Source: CAD feature listing. Evaluate the final solid. Frame: model axes, mm. A direction names the side the tool comes from. Give positions to 0.01 mm unless a question says otherwise; leave off trailing zeros. Write each loop counter-clockwise with the first axis right and the second up, starting at its lowest first coordinate (ties: lowest second). Pieces come first, ordered by that corner, then holes. Notation, with made-up numbers: M 49,1.5 L 84,1.5 A28 cw 84,21.5 Z; hole C 40,41 d9. An arc over 180 degrees is marked long. Use CSV: the item, a comma, the result in double quotes. Start each with the question number.
from build123d import *

# Parameters (mm, degrees)
BOSS_EXTRUDE1_DEPTH = 6
BOSS_EXTRUDE2_START = 6
BOSS_EXTRUDE2_DEPTH = 6
BOSS_EXTRUDE3_DEPTH = 1.5
CUT_EXTRUDE3_DEPTH  = 6
CHAMFER1_SIZE       = 0.858848527
CHAMFER1_SIZE_2     = 1
CHAMFER2_SIZE       = 1


with BuildPart() as part:
    # Sketch3 → Boss-Extrude1 (new body)
    with BuildSketch(Plane.XY):
        with BuildLine():
            Line((3.263957589, 12.181255556), (-159.230871571, 55.721613803))
            ThreePointArc((-159.230871571, 55.721613803), (-167.389036276, 0), (-159.230871571, -55.721613803))
            Line((-159.230871571, -55.721613803), (-83.597968128, -35.455838404))
            Line((-83.597968128, -35.455838404), (3.263957589, -12.181255556))
            ThreePointArc((3.263957589, -12.181255556), (12.610963724, 0), (3.263957589, 12.181255556))
        make_face()
    extrude(amount=BOSS_EXTRUDE1_DEPTH)

    # Sketch3<3> → Boss-Extrude2 (add)
    with BuildSketch(Plane.XY.offset(BOSS_EXTRUDE2_START)):
        with BuildLine():
            ThreePointArc((3.263957589, -12.181255556), (12.610963724, 0), (3.263957589, 12.181255556))
            Line((3.263957589, 12.181255556), (-159.230871571, 55.721613803))
            ThreePointArc((-159.230871571, 55.721613803), (-167.389036276, 0), (-159.230871571, -55.721613803))
            Line((-159.230871571, -55.721613803), (-83.597968128, -35.455838404))
            Line((-83.597968128, -35.455838404), (3.263957589, -12.181255556))
        make_face()
        with BuildLine():
            Line((-85.282065581, -29.695433875), (-155.066564747, -48.39413407))
            ThreePointArc((-155.066564747, -48.39413407), (-161.389036276, 0), (-155.066564747, 48.39413407))
            Line((-155.066564747, 48.39413407), (-85.282065581, 29.695433875))
            ThreePointArc((-85.282065581, 29.695433875), (-89.143036276, 0), (-85.282065581, -29.695433875))
        make_face(mode=Mode.SUBTRACT)
        with BuildLine():
            Line((1.711043318, -6.385700598), (-79.486479098, -28.142511157))
            ThreePointArc((-79.486479098, -28.142511157), (-83.143036276, 0), (-79.486479098, 28.142511157))
            Line((-79.486479098, 28.142511157), (1.711043318, 6.385700598))
            ThreePointArc((1.711043318, 6.385700598), (6.610963724, 0), (1.711043318, -6.385700598))
        make_face(mode=Mode.SUBTRACT)
    extrude(amount=BOSS_EXTRUDE2_DEPTH)

    # Sketch4 → Boss-Extrude3 (add)
    with BuildSketch(Plane.XY.offset(6)):
        with BuildLine():
            ThreePointArc((-79.486479098, 28.142511157), (-80.363791639, 24.584864194), (-81.12226241, 21))
            Line((-81.12226241, 21), (-52.830264568, 21))
            Line((-52.830264568, 21), (-79.486479098, 28.142511157))
        make_face()
        with BuildLine():
            Line((-79.486479098, -28.142511157), (-52.830264568, -21))
            Line((-52.830264568, -21), (-81.12226241, -21))
            ThreePointArc((-81.12226241, -21), (-80.363791639, -24.584864194), (-79.486479098, -28.142511157))
        make_face()
        with BuildLine():
            Line((-48.09821376, 19.732050808), (-48.09821376, -19.732050808))
            Line((-48.09821376, -19.732050808), (1.711043318, -6.385700598))
            ThreePointArc((1.711043318, -6.385700598), (6.610963724, 0), (1.711043318, 6.385700598))
            Line((1.711043318, 6.385700598), (-48.09821376, 19.732050808))
        make_face()
    extrude(amount=BOSS_EXTRUDE3_DEPTH)

    # Sketch5 → Cut-Extrude3 (cut)
    with BuildSketch(Plane.XY.offset(6)):
        with BuildLine():
            Line((-81.12226241, 21), (-87.228470489, 21))
            ThreePointArc((-87.228470489, 21), (-89.143036276, 0), (-87.228470489, -21))
            Line((-87.228470489, -21), (-81.12226241, -21))
            ThreePointArc((-81.12226241, -21), (-83.143036276, 0), (-81.12226241, 21))
        make_face()
    extrude(amount=CUT_EXTRUDE3_DEPTH, mode=Mode.SUBTRACT)

    # Chamfer1
    # the kernel refuses this chamfer: 1, 0.858848527 mm, written as the material it takes off along each edge
    with BuildSketch(Plane(origin=(-87.228470489, 21, 6), x_dir=(0.1850514416549976, 0.9827288354075131, 0), z_dir=(0, 0, 1))) as chamfer1_piece_1:
        with BuildLine():
            Line((0.995740125, 0), (CHAMFER1_SIZE * 0.185051441724, -CHAMFER1_SIZE * 0.982728835776))
            Line((CHAMFER1_SIZE * 0.185051441724, -CHAMFER1_SIZE * 0.982728835776), (0, 0))
            ThreePointArc((0, 0), (0.511949844, 0.001066408), (0.995740125, 0))
        make_face()
    extrude(amount=8.560742024, mode=Mode.SUBTRACT)
    with BuildSketch(Plane(origin=(-87.228470489, -21, 6), x_dir=(1, 0, 0), z_dir=(0, 0, 1))) as chamfer1_piece_2:
        with BuildLine():
            Line((CHAMFER1_SIZE_2, 0), (0.158025015, -0.841974985))
            ThreePointArc((0.158025015, -0.841974985), (0.080319075, -0.432228603), (0, 0))
            Line((0, 0), (CHAMFER1_SIZE_2, 0))
        make_face()
    extrude(amount=8.571682988, mode=Mode.SUBTRACT)

    # Chamfer2
    chamfer2_edges = [part.edges().sort_by_distance(p)[0] for p in [
        (-86.244364999, -25.784214234, 12),
        (-83.67536645, -21, 12),
        (-86.706914653, 21.489271267, 12),
        (-86.649457982, -21.420987493, 12),
        (-86.228906055, 25.852006602, 12),
        (-120.174315164, -39.044783972, 12),
        (12.610963724, 0, 12),
        (-167.389036276, 0, 12),
        (-38.88771789, 17.264105877, 12),
        (-38.88771789, -17.264105877, 12),
        (-77.983456991, 33.951434679, 12),
        (-77.983456991, -33.951434679, 12),
        (-120.174315164, 39.044783972, 12),
        (-161.389036276, 0, 12),
        (6.610963724, 0, 12),
        (-80.363791639, 24.584864194, 12),
        (-80.363791639, -24.584864194, 12),
        (-83.745942186, 21, 12),
    ]]
    chamfer(chamfer2_edges, length=CHAMFER2_SIZE)


solid = part.part
Item 1: Section C-C (x = -73). Return the cut outline in (y, z), plus the area to 3 significant figures.
Item 2: Section D-D (x = -101.5). Return the cut outline in (y, z).
Item 3: Pull-direction query (X, two-part tool) for faces 1 (the flat face through (-84, -24, 12)), 2 (the flat face through (-27, 0, 7.5)), 3 (the flat face through (-76.97, 33.17, 11.49)); classes: released by +X, released by -X, zero draft, split by the parting line, or undercut.
Item 4: Section A-A (x = -142.5). Return the cut outline in (y, z), plus the area to 3 significant figures.
Item 5: Material intervals for probe 1 along Z at (x, y) = (-91, 7.5); probe 2 along Y at (x, z) = (-55, 11.75); probe 3 along Y at (x, z) = (2.5, 8.5), sorted ascending.
Item 6: Section B-B (z = 2). Return the cut outline in (x, y), plus the area to 3 significant figures.
Item 7: Set-up query: faces 4 (the conical face through (-166.56, 0.79, 11.83)), 5 (the cylindrical face through (-86.257, -25.729, 8.465)). Return all of +Z, -Z, +X, -X, +Y, -Y with unobstructed straight access to the full face (end or side cutting, diameter ignored); none if empty.
Item 8: Contact query for flat-ended pins moving along their axis: pin 1 Ø4 at (y, z) = (8, 7.5) entering from +X; pin 2 Ø2.5 at (x, z) = (-74.5, 8.5) entering from -Y; pin 3 Ø2 at (x, z) = (-132, 9) entering from -Y. Output: stop coordinate, or through.
Output values:
1,outline,"M -32.62,0 L 32.62,0 L 32.62,11 L 31.58,12 L 27.44,12 L 26.4,11 L 26.4,7.5 L 21,7.5 L 21,6 L -21,6 L -21,7.5 L -26.4,7.5 L -26.4,11 L -27.44,12 L -31.58,12 L -32.62,11 Z"
1,area,"480 mm2"
2,outline,"M -40.25,0 L 40.25,0 L 40.25,11 L 39.22,12 L 35.08,12 L 34.04,11 L 34.04,6 L -34.04,6 L -34.04,11 L -35.08,12 L -39.22,12 L -40.25,11 Z"
3,face 1,"zero draft"
3,face 2,"undercut"
3,face 3,"released by +X"
4,outline,"M -51.24,0 L 51.24,0 L 51.24,11 L 50.2,12 L 46.06,12 L 45.03,11 L 45.03,6 L -45.03,6 L -45.03,11 L -46.06,12 L -50.2,12 L -51.24,11 Z"
4,area,"687 mm2"
5,probe 1,"z = 0 to 6"
5,probe 2,"y = -27.02 to -22.36, 22.36 to 27.02"
5,probe 3,"y = -12.39 to -6.12, 6.12 to 12.39"
6,outline,"M -159.23,-55.72 L 3.26,-12.18 A12.61 ccw 3.26,12.18 L -159.23,55.72 A194.37 ccw Z"
6,area,"11,800 mm2"
7,face 4,"+Z, -X"
7,face 5,"+Z"
8,pin 1,"stops at x = 11.09"
8,pin 2,"stops at y = -33.35"
8,pin 3,"stops at y = -48.69"
